Build history of the part. All positions in model axes, mm. Face numbers are marked on the shaded views. A direction names the side the tool comes from. Round coordinates to 2 decimals unless told otherwise and drop trailing zeros. Loops run counter-clockwise (first coordinate to the right, second up) from the corner with the lowest first, then second, coordinate; pieces in that order, holes last. Notation, with made-up numbers: (-14, 52) -> (-1, 52) arc R10 ccw to (-1, 68) -> close; hole circle Ø2 at (75, -16.5). An arc over 180 degrees is marked (long way). Put each result on its own line as item: value. Start each with the question number.
Item 1: Tool access for the marked faces 1, 2, 3 and 4: list every direction of +Z, -Z, +X, -X, +Y, -Y with a clear straight run to the whole face (end or side of a thin tool).
Item 2: Cut at D-D, the plane z = 3. List the corners of the cut face in (x, y), plus the area to 3 significant figures.
Item 3: Cut at A-A, the plane y = 9. List the corners of the cut face in (x, z), plus the area to 3 significant figures.
Item 4: Cut at C-C, the plane y = -11. List the corners of the cut face in (x, z).
Item 5: Flat gauge pins, fed straight in: pin 1 Ø6 at (x, y) = (47.5, 10.5) entering from -Z; pin 2 Ø3 at (x, y) = (7.6, -5) entering from +Z; pin 3 Ø1.5 at (x, z) = (14.5, 5.5) entering from -Y; pin 4 Ø1.5 at (x, y) = (7.6, -15) entering from +Z. Where does each tip first touch, or does it go through?
Item 6: Drill centre lines: probe 1 along Y at (x, z) = (7.6, 3.75); probe 2 along Y at (x, z) = (42.5, 30.3); probe 3 along Y at (x, z) = (34, 17.5). Where is each one in solid material? Low to high. Write a range as [from, to].
Item 7: Cut at B-B, the plane x = 37.5. List the corners of the cut face in (y, z), plus the area to 3 significant figures.
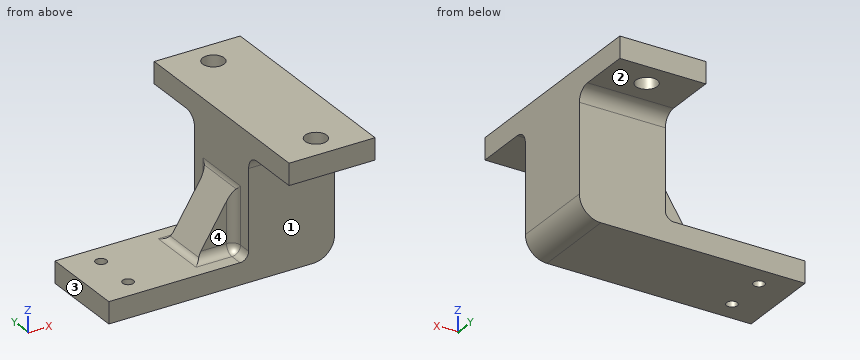
```python
from build123d import *

# Parameters (mm, degrees)
SKETCH_1_W          = 52.5
SKETCH_1_H          = 20
SKETCH_1_R          = 1.27
SKETCH_1_R_2        = 1.25
EXTRUDE_1_DEPTH     = 5
SKETCH_2_W          = 20
SKETCH_2_H          = 20
EXTRUDE_2_DEPTH     = 28.5
SKETCH_4_W          = 20
SKETCH_4_H          = 5
EXTRUDE_3_DEPTH     = 25
SKETCH_5_R          = 2.5
CUT_EXTRUDE_1_DEPTH = 18
FILLET_1_R          = 3
RIB_1_REACH         = 69.108
SKETCH_6_WALL_W     = 153.524907632
SKETCH_6_WALL_H     = 10
FILLET_2_R          = 5
FILLET_3_R          = 2


with BuildPart() as part:
    # 草图1 → 凸台-拉伸1 (new body)
    with BuildSketch(Plane.XY):
        with Locations((26.25, -10)):
            Rectangle(SKETCH_1_W, SKETCH_1_H)
        with Locations((7.6, -5)):
            Circle(SKETCH_1_R, mode=Mode.SUBTRACT)
        with Locations((7.6, -15)):
            Circle(SKETCH_1_R_2, mode=Mode.SUBTRACT)
    extrude(amount=EXTRUDE_1_DEPTH)

    # 草图2 → 凸台-拉伸2 (add)
    with BuildSketch(Plane.XY.offset(5)):
        with Locations((42.5, -10)):
            Rectangle(SKETCH_2_W, SKETCH_2_H)
    extrude(amount=EXTRUDE_2_DEPTH)

    # 草图4 → 凸台-拉伸3 (add, symmetric)
    with BuildSketch(Plane(origin=(0, -10, 0), x_dir=(1, 0, 0), z_dir=(0, 1, 0))):
        with Locations((42.5, -31)):
            Rectangle(SKETCH_4_W, SKETCH_4_H)
    extrude(amount=EXTRUDE_3_DEPTH, both=True)

    # 草图5 → 切除-拉伸1 (cut, symmetric)
    with BuildSketch(Plane.XY.offset(33.5)):
        with Locations((42.5, 9)):
            Circle(SKETCH_5_R)
        with Locations((42.5, -29)):
            Circle(SKETCH_5_R)
    extrude(amount=CUT_EXTRUDE_1_DEPTH, both=True, mode=Mode.SUBTRACT)

    # 圆角1
    fillet_1_edges = [part.edges().sort_by_distance(p)[0] for p in [
        (42.5, -20, 28.5),
        (42.5, 0, 28.5),
    ]]
    fillet(fillet_1_edges, radius=FILLET_1_R)

    # 草图6 wall → 筋1 (add, up to next)
    with BuildSketch(Plane(origin=(27.883344013, -10, 12.320105985), x_dir=(0.533450292048, 0, 0.845831416959), z_dir=(0.845831416959, 0, -0.533450292048)), mode=Mode.PRIVATE) as rib_1_sk1:
        Rectangle(SKETCH_6_WALL_W, SKETCH_6_WALL_H)
    rib_1_tool1 = extrude(rib_1_sk1.sketch, amount=RIB_1_REACH, mode=Mode.PRIVATE) - part.part
    add(rib_1_tool1.solids().sort_by_distance((27.883344013, -10, 12.320105985))[0])

    # 圆角2
    fillet_2_edges = [part.edges().sort_by_distance(p)[0] for p in [
        (52.5, -10, 0),
    ]]
    fillet(fillet_2_edges, radius=FILLET_2_R)

    # 圆角3
    fillet_3_edges = [part.edges().sort_by_distance(p)[0] for p in [
        (32.5, -2.5, 5),
        (32.5, -17.5, 5),
        (23.266688025, -10, 5),
        (32.5, -5, 12.320105985),
        (27.883344013, -15, 5),
        (32.5, -10, 19.640211969),
        (27.883344013, -5, 5),
        (32.5, -15, 12.320105985),
    ]]
    fillet(fillet_3_edges, radius=FILLET_3_R)


solid = part.part
```
Reply:
1. face 1: -Z, +X, -X, -Y
1. face 2: -Z, +X, -X, +Y
1. face 3: +Z, -Z, -X, +Y, -Y
1. face 4: +Z, -X, -Y
2. outline: (0, -20) -> (52.08, -20) -> (52.08, 0) -> (0, 0) -> close; hole circle Ø2.54 at (7.6, -5); hole circle Ø2.5 at (7.6, -15)
2. area: 1,030 mm^2
3. outline: (32.5, 28.5) -> (40, 28.5) -> (40, 33.5) -> (32.5, 33.5) -> close; (45, 28.5) -> (52.5, 28.5) -> (52.5, 33.5) -> (45, 33.5) -> close
3. area: 75.0 mm^2
4. outline: (0, 0) -> (47.5, 0) arc R5 ccw to (52.5, 5) -> (52.5, 33.5) -> (32.5, 33.5) -> (32.5, 20.22) arc R2 cw to (32.19, 19.15) -> (23.86, 5.93) arc R2 cw to (22.16, 5) -> (0, 5) -> close
5. pin 1: stops at z = 28.5
5. pin 2: stops at z = 5
5. pin 3: stops at y = -20
5. pin 4: passes through
6. probe 1: y = [-20, -16.25], [-13.75, -6.27], [-3.73, 0]
6. probe 2: y = [-35, -31.5], [-26.5, 6.5], [11.5, 15]
6. probe 3: y = [-20, 0]
7. outline: (-35, 28.5) -> (-23, 28.5) arc R3 cw to (-20, 25.5) -> (-20, 0) -> (0, 0) -> (0, 25.5) arc R3 cw to (3, 28.5) -> (15, 28.5) -> (15, 33.5) -> (-35, 33.5) -> close
7. area: 824 mm^2
